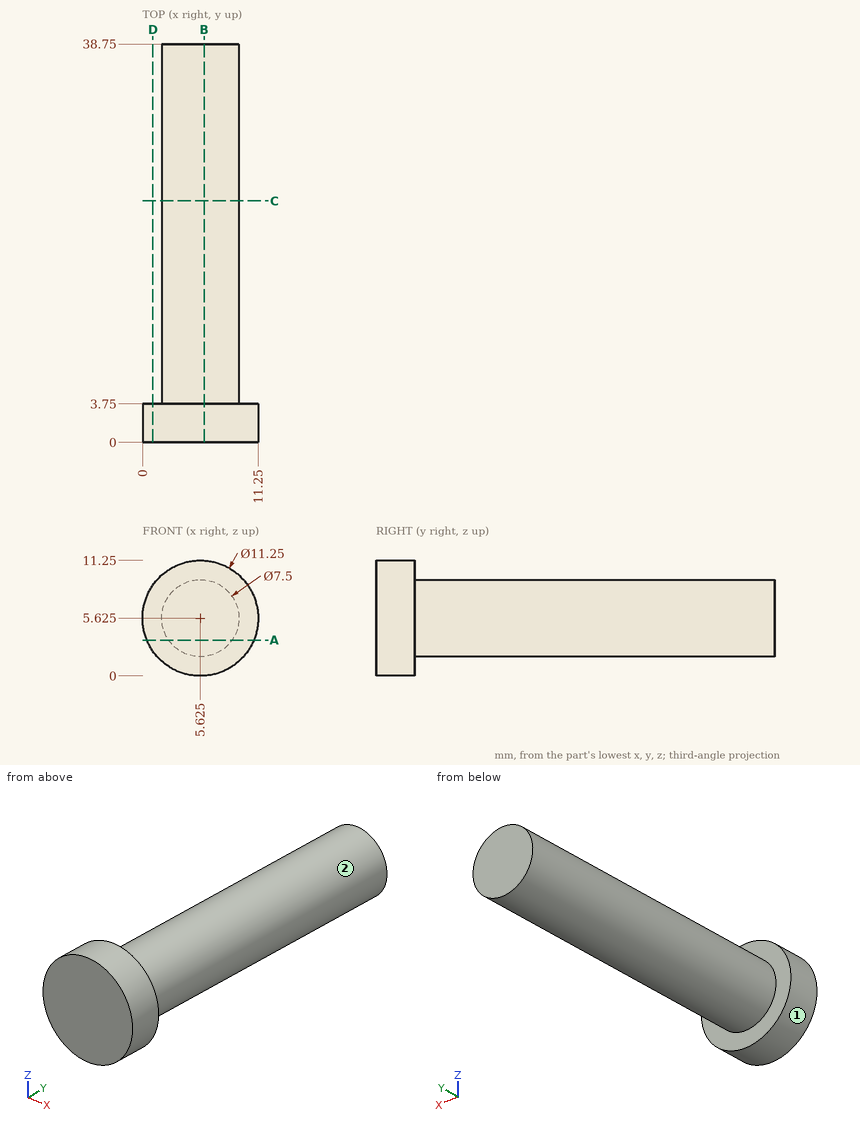
For this review, use the dimensioned drawing (mm, ordinates from the lowest corner) and the shaded views. A direction names the side the tool comes from. Give positions to 0.01 mm unless a question says otherwise; leave off trailing zeros. Loops run counter-clockwise (first coordinate to the right, second up) from the corner with the lowest first, then second, coordinate; pieces in that order, holes last. Notation, with made-up numbers: (-38, -5.5) -> (-3, -5.5) arc R15 cw to (-3, 2.5) -> close; hole circle Ø11 at (2, 11). An arc over 180 degrees is marked (long way). One line per question, with ' | ' between items. Start each with the question number.
(1) For line 1 (Y direction, x = 7.5, z = 1); line 2 (Z direction, x = 5.75, y = 12); line 3 (X direction, y = 11, z = 2.25), list the stretches that pass through material, from the lowest coordinate up.
(2) Insertion check: P1, Ø4, axis at y = 26.5, z = 4, coming from the -X side (3 decimals); P2, Ø5, axis at x = 3.5, y = 29, coming from the +Z side (3 decimals); P3, Ø1, axis at x = 4, z = 10, coming from the +Y side. Each pin has a flat end and moves straight along its axis. Give the tip position at first contact, or say it passes through.
(3) We need section A-A (z = 3.5). State the section outline as (x, y) points, and give its area (3 significant figures).
(4) We need section B-B (x = 6). State the section outline as (y, z) points.
(5) We need section C-C (y = 23.5). State the section outline as (x, z) points (3 decimals).
(6) For the marked faces 1 and 2, list the 3-axis set-ups (+Z, -Z, +X, -X, +Y, -Y) from which the entire face can be reached by the end or side of a thin tool; tool diameter is ignored.
(7) We need section D-D (x = 1). State the section outline as (y, z) points.
The answers:
1) line 1: y = 0 to 3.75 | line 2: z = 1.88 to 9.37 | line 3: x = 3.99 to 7.26
2) P1: stops at x = 1.875 | P2: stops at z = 9.375 | P3: stops at y = 3.75
3) outline: (0.42, 0) -> (10.83, 0) -> (10.83, 3.75) -> (8.71, 3.75) -> (8.71, 38.75) -> (2.54, 38.75) -> (2.54, 3.75) -> (0.42, 3.75) -> close | area: 255 mm^2
4) outline: (0, 0.01) -> (3.75, 0.01) -> (3.75, 1.89) -> (38.75, 1.89) -> (38.75, 9.36) -> (3.75, 9.36) -> (3.75, 11.24) -> (0, 11.24) -> close
5) outline: circle Ø7.5 at (5.625, 5.625)
6) face 1: +Y, -Y | face 2: +Y
7) outline: (0, 2.42) -> (3.75, 2.42) -> (3.75, 8.83) -> (0, 8.83) -> close
